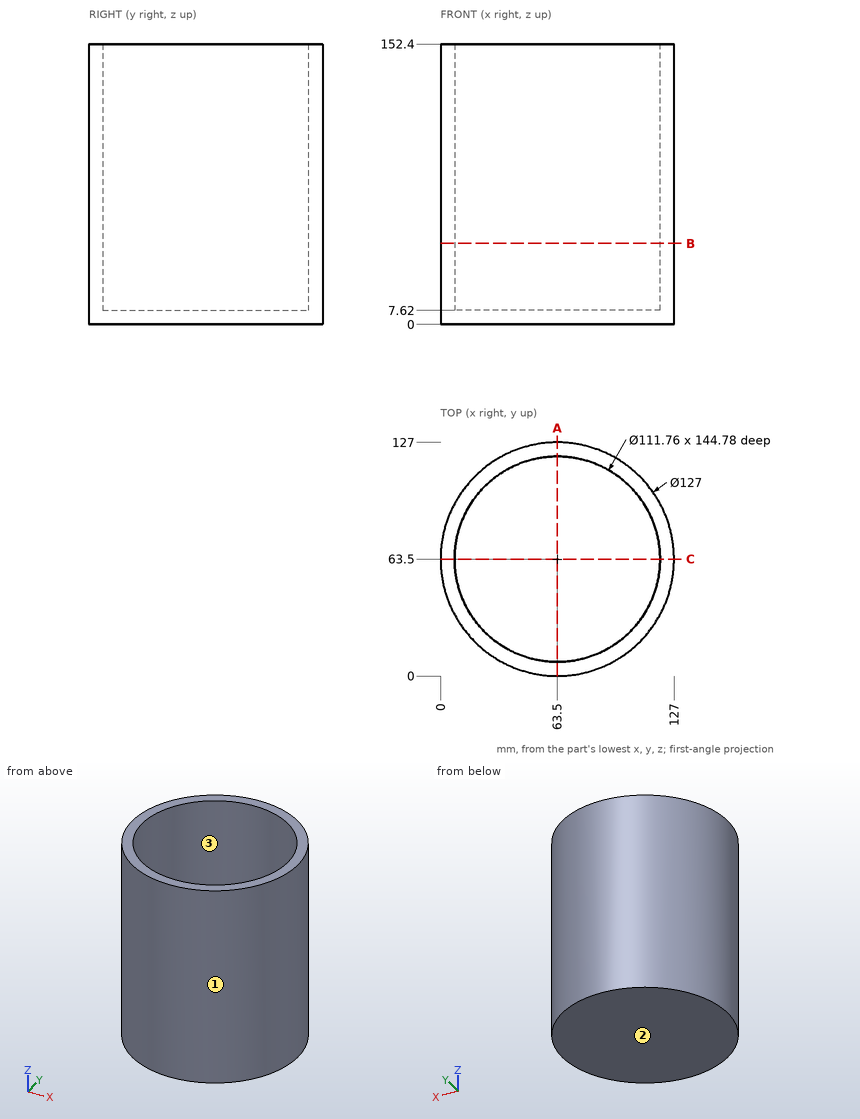
Here's the drawing with two shaded views (mm, measured from the low corner). I have some questions. Round coordinates to 2 decimals unless told otherwise and drop trailing zeros. Write each loop counter-clockwise with the first axis right and the second up, starting at its lowest first coordinate (ties: lowest second). Pieces come first, ordered by that corner, then holes. Notation, with made-up numbers: M 69.25,11.5 L 96.25,11.5 A20 cw 96.25,36.5 Z; hole C 76,-28.75 d11. An arc over 180 degrees is marked long. Write each question's results on one line, items separated by ' | '. Start each with the question number.
1. I'm going to push flat-ended pins straight in: pin 1 Ø12 at (x, y) = (48.5, 45.5) entering from +Z; pin 2 Ø12 at (y, z) = (34, 79) entering from -X; pin 3 Ø4 at (x, z) = (90, 82) entering from +Y; pin 4 Ø6 at (x, y) = (78.5, 37.5) entering from -Z. Where does each tip first touch, or does it pass through?
2. I need wall thicknesses on L1, parallel to Y at x = 63.5, z = 99; L2, parallel to Z at x = 36.5, y = 36.5. Which ranges of each line are inside material? Lowest first, please. Write a range as from..to.
3. Imagine slicing it at A-A on x = 63.5. List the corners of the cut face in (y, z) for me, and give its area (3 significant figures).
4. Thinking about a two-plate mould opening in Y: for the marked faces 1, 2 and 3, which applies, +Y half, -Y half, draft (parallel to the pull), parting line (faces both ways), or undercut?
5. Imagine slicing it at B-B on z = 44. List the corners of the cut face in (x, y) for me, and give its area (3 significant figures).
Result sheet:
1) pin 1: stops at z = 7.62 | pin 2: stops at x = 4.51 | pin 3: stops at y = 122.08 | pin 4: stops at z = 0
2) L1: y = 0..7.62, 119.38..127 | L2: z = 0..7.62
3) outline: M 0,0 L 127,0 L 127,152.4 L 119.38,152.4 L 119.38,7.62 L 7.62,7.62 L 7.62,152.4 L 0,152.4 Z | area: 3,170 mm^2
4) face 1: parting line | face 2: draft | face 3: undercut
5) outline: C 63.5,63.5 d127; hole C 63.5,63.5 d111.76 | area: 2,860 mm^2
